from build123d import *

# Parameters (mm, degrees)
F0_W     = 45.4592518508
F0_H     = 59.5056191087
F0_W_2   = 45.7147136331
F0_H_2   = 116.1159910262
F1_DEPTH = 38.608
F2_W     = 45.6728860736
F2_H     = 59.5056191087
F3_DEPTH = 35.306
F5_W     = 33.7057895958
F5_H     = 34.315392375
F5_H_2   = 34.9249877036
F5_W_2   = 33.7739177048
F6_DEPTH = 30.734
F8_DEPTH = 29.21


with BuildPart() as f1:
    # F0 (on Top) → F1 (new body)
    with BuildSketch(Plane.XY):
        Polygon((-27.5232736021, 56.6103719175), (-77.1979466081, 56.6103719175), (-77.1979466081, -59.5056191087), (-27.5232736021, -59.5056191087), (-27.5232736021, 0), align=None)
        with Locations((-4.7936476767, -29.7528095543)):
            Rectangle(F0_W, F0_H)
        with Locations((-100.0553034246, -1.4476235956)):
            Rectangle(F0_W_2, F0_H_2)
    extrude(amount=F1_DEPTH)

    # F2 (on face) → F3 (join)
    with BuildSketch(Plane.XY.offset(38.608)):
        with Locations((-100.0762172043, -29.7528095543)):
            Rectangle(F2_W, F2_H)
    extrude(amount=F3_DEPTH)


with BuildPart() as f6:
    # F5 (on Top) → F6 (new body)
    with BuildSketch(Plane.XY):
        Polygon((-34.2192724347, 0), (0, 0), (0, 34.9249877036), (0, 35.2751240134), (-34.2192724347, 35.2751240134), align=None)
        Polygon((0, -34.315392375), (0, 0), (-34.2192724347, 0), (-34.315392375, 0), (-34.315392375, -34.315392375), align=None)
        with Locations((16.8528947979, -17.1576961875)):
            Rectangle(F5_W, F5_H)
        with Locations((16.8528947979, 17.4624938518)):
            Rectangle(F5_W, F5_H_2)
        with Locations((50.5927484483, 17.4624938518)):
            Rectangle(F5_W_2, F5_H_2)
    extrude(amount=F6_DEPTH)

    # F7 (on face) → F8 (join)
    with BuildSketch(Plane.XY.offset(30.734)):
        Polygon((0, 35.2751240134), (-34.2192724347, 35.2751240134), (-34.2192724347, 0), (0, 0), (0, 34.9249877036), align=None)
    extrude(amount=F8_DEPTH)


solid = f6.part
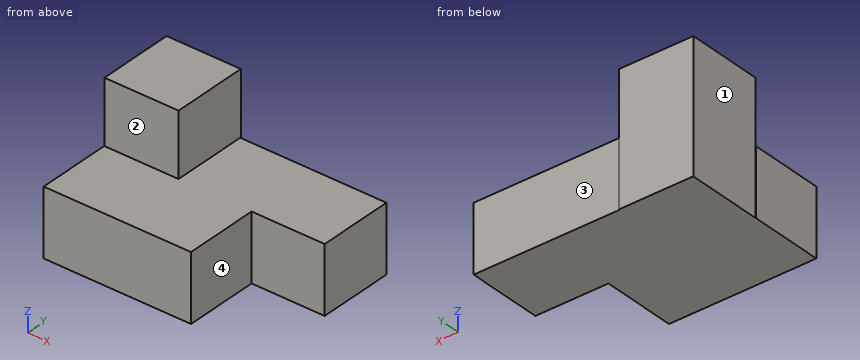
The listing builds one solid part. Answer for the finished solid, in the listing's coordinates (mm). Face numbers are marked on the shaded views. A direction names the side the tool comes from. Coordinates: 2 decimals unless noted, no trailing zeros. Loops run counter-clockwise (first coordinate to the right, second up) from the corner with the lowest first, then second, coordinate; pieces in that order, holes last. Notation, with made-up numbers: (33, 58) -> (44, 58) arc R25 ccw to (44, 71) -> close; hole circle Ø11 at (67.25, 83). An arc over 180 degrees is marked (long way). Answer in a Markdown table with one row per item. Add a question column.
1. The part is cut by section D-D, the plane z = 42. Write down the section's boundary in (x, y).
2. The part is cut by section C-C, the plane x = -16.5. Write down the section's boundary in (y, z), then the cut area to 3 significant figures.
3. The part is cut by section A-A, the plane z = 29.5. Write down the section's boundary in (x, y).
4. Consider line 1 (X direction, y = 19.5, z = 56.5); line 2 (X direction, y = -19.5, z = 25); line 3 (Y direction, x = 44, z = 18.5). Determine where each line is inside the solid, lowest interval first. Write a range as [from, to].
5. The part is cut by section B-B, the plane y = 15. Write down the section's boundary in (x, z), then the cut area to 3 significant figures.
6. Flat-ended cylindrical pins translate along their axes: P1, Ø6, axis at x = 13, z = 22, coming from the +Y side (3 decimals); P2, Ø6, axis at y = 3.5, z = 35.5, coming from the -X side; P3, Ø9, axis at y = -22, z = 17, coming from the +X side. Find the tip coordinate at first contact, or state that the pin passes through.
7. For the marked faces 1, 2, 3 and 4, determine the directions among +Z, -Z, +X, -X, +Y, -Y from which every point of the face is accessible in a straight line to the end or side of a thin tool.
Answer below:
| question | item | result |
|---|---|---|
| 1 | outline | (-34.22, 0) -> (0, 0) -> (0, 35.28) -> (-34.22, 35.28) -> close |
| 2 | outline | (-34.32, 0) -> (35.28, 0) -> (35.28, 59.94) -> (0, 59.94) -> (0, 30.73) -> (-34.32, 30.73) -> close |
| 2 | area | 3,170 mm2 |
| 3 | outline | (-34.32, -34.32) -> (33.71, -34.32) -> (33.71, 0) -> (67.48, 0) -> (67.48, 34.92) -> (0, 34.92) -> (0, 35.28) -> (-34.22, 35.28) -> (-34.22, 0) -> (-34.32, 0) -> close |
| 4 | line 1 | [-34.22, 0] |
| 4 | line 2 | [-34.32, 33.71] |
| 4 | line 3 | [0, 34.92] |
| 5 | outline | (-34.22, 0) -> (67.48, 0) -> (67.48, 30.73) -> (0, 30.73) -> (0, 59.94) -> (-34.22, 59.94) -> close |
| 5 | area | 4,130 mm2 |
| 6 | P1 | y = 34.925 |
| 6 | P2 | x = -34.22 |
| 6 | P3 | x = 33.71 |
| 7 | face 1 | +Z, -Z, -X, +Y |
| 7 | face 2 | +Z, +X, -X, -Y |
| 7 | face 3 | +Z, -Z, +X, +Y |
| 7 | face 4 | +Z, -Z, +X, -Y |
